CAD build for the part. Positions are in the model's coordinates, mm. Coordinates: 2 decimals unless noted, no trailing zeros. Loops run counter-clockwise (first coordinate to the right, second up) from the corner with the lowest first, then second, coordinate; pieces in that order, holes last.
1) Wall check: line 1 along X through (y, z) = (25.5, -5.25); line 2 along X through (y, z) = (37.5, -11); line 3 along Y through (x, z) = (6, -8.25). Give the ranges that are in metal, low to high.
2) Saw through at A-A, the plane z = -6.5. Give the number of separate pieces and of enclosed holes in the cut face, and give its area (3 significant figures).
3) Saw through at B-B, the plane y = 25.4. Write the cut outline in (x, z), and give its area (3 significant figures).
4) Pin check, flat tip, straight feed: pin 1 Ø4 at (x, y) = (12.7, 38.1) entering from +Z. Stop position of the tip, or through.
```python
from build123d import *

# Parameters (mm, degrees)
SKETCH2_W           = 50.8
SKETCH2_H           = 160.02
BOSS_EXTRUDE1_DEPTH = 12.7
SKETCH3_R           = 2.4892
CUT_EXTRUDE1_DEPTH  = 169.369624339
FILLET1_R           = 6.35


with BuildPart() as part:
    # Sketch2 → Boss-Extrude1 (new body)
    with BuildSketch(Plane.XY):
        with Locations((25.4, 80.01)):
            Rectangle(SKETCH2_W, SKETCH2_H)
    extrude(amount=-BOSS_EXTRUDE1_DEPTH)

    # Sketch3 → Cut-Extrude1 (cut, through all)
    with BuildSketch(Plane.XY):
        with Locations((12.7, 147.32)):
            Circle(SKETCH3_R)
        with Locations((38.1, 147.32)):
            Circle(SKETCH3_R)
        with Locations((12.7, 114.3)):
            Circle(SKETCH3_R)
        with Locations((12.7, 101.6)):
            Circle(SKETCH3_R)
        with Locations((12.7, 88.9)):
            Circle(SKETCH3_R)
        with Locations((12.7, 76.2)):
            Circle(SKETCH3_R)
        with Locations((12.7, 63.5)):
            Circle(SKETCH3_R)
        with Locations((12.7, 50.8)):
            Circle(SKETCH3_R)
        with Locations((12.7, 38.1)):
            Circle(SKETCH3_R)
        with Locations((12.7, 25.4)):
            Circle(SKETCH3_R)
        with Locations((12.7, 12.7)):
            Circle(SKETCH3_R)
        with Locations((38.1, 101.6)):
            Circle(SKETCH3_R)
        with Locations((38.1, 88.9)):
            Circle(SKETCH3_R)
        with Locations((38.1, 76.2)):
            Circle(SKETCH3_R)
        with Locations((38.1, 63.5)):
            Circle(SKETCH3_R)
        with Locations((38.1, 50.8)):
            Circle(SKETCH3_R)
        with Locations((38.1, 38.1)):
            Circle(SKETCH3_R)
        with Locations((38.1, 25.4)):
            Circle(SKETCH3_R)
        with Locations((38.1, 12.7)):
            Circle(SKETCH3_R)
        with Locations((38.1, 114.3)):
            Circle(SKETCH3_R)
    extrude(amount=-CUT_EXTRUDE1_DEPTH, mode=Mode.SUBTRACT)

    # Fillet1
    fillet1_edges = [part.edges().sort_by_distance(p)[0] for p in [
        (0, 160.02, -6.35),
        (50.8, 160.02, -6.35),
        (50.8, 0, -6.35),
        (0, 0, -6.35),
    ]]
    fillet(fillet1_edges, radius=FILLET1_R)


solid = part.part
```
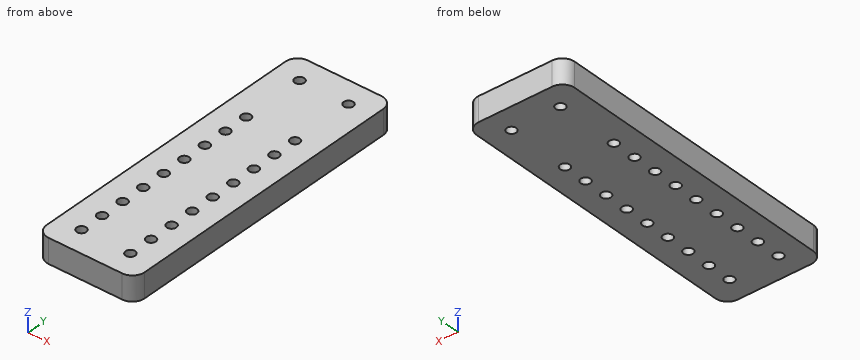
Data:
1. line 1: x = 0 to 10.21, 15.19 to 35.61, 40.59 to 50.8
1. line 2: x = 0 to 10.28, 15.12 to 35.68, 40.52 to 50.8
1. line 3: y = 0.01 to 160.01
2. separate pieces: 1
2. enclosed holes: 20
2. area: 7,710 mm2
3. outline: (0, -12.7) - (10.21, -12.7) - (10.21, 0) - (0, 0) - close; (15.19, -12.7) - (35.61, -12.7) - (35.61, 0) - (15.19, 0) - close; (40.59, -12.7) - (50.8, -12.7) - (50.8, 0) - (40.59, 0) - close
3. area: 519 mm2
4. pin 1: passes through
